Part print with two shaded views. Sizes in mm from the minimum x, y, z corner. A direction names the side the tool comes from. Round coordinates to 2 decimals unless told otherwise and drop trailing zeros. Write each loop counter-clockwise with the first axis right and the second up, starting at its lowest first coordinate (ties: lowest second). Pieces come first, ordered by that corner, then holes.
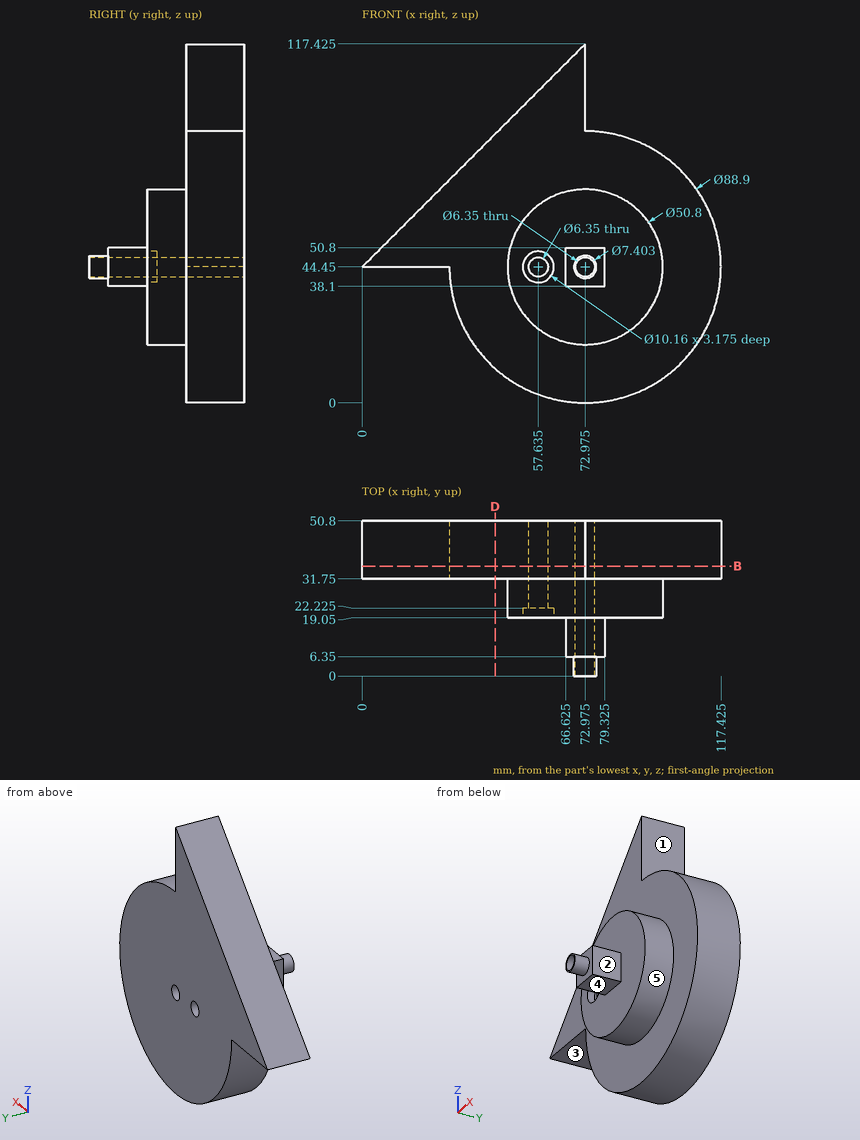
Q1. Drop flat-ended pins along their axis: pin 1 (8 mm diameter, centred on x = 74.5, z = 27, fed in from -Y); pin 2 (10 mm diameter, centred on y = 11.5, z = 47, fed in from +X) (1 decimal); pin 3 (10 mm diameter, centred on x = 70, y = 15, fed in from -Z). Give the stop position or say it passes through.
Values follow:
pin 1: stops at y = 19.05
pin 2: stops at x = 79.3
pin 3: stops at z = 19.05
Q2. Cut at B-B on y = 36. State how many separate pieces and enclosed holes the cut face has.
Values follow:
separate pieces: 1
enclosed holes: 2
Q3. Wall check: L1, parallel to X at y = 25, z = 44; L2, parallel to X at y = 47.5, z = 42 (1 decimal); L3, parallel to Y at x = 90.5, z = 10. Give the ranges that are in metal, low to high.
Values follow:
L1: x = 47.58 to 54.49, 60.78 to 69.83, 76.12 to 98.37
L2: x = 28.6 to 55.6, 59.7 to 71, 75 to 117.4
L3: y = 31.75 to 50.8
Q4. Cut at D-D on x = 43.5. Write the cut outline in (y, z), plus the area to 3 significant figures.
Values follow:
outline: (31.75, 11.18) - (50.8, 11.18) - (50.8, 87.95) - (31.75, 87.95) - close
area: 1,460 mm2
Q5. Which spindle directions (+Z, -Z, +X, -X, +Y, -Y) get a long thin tool onto all of the face, cutting with end or side? Do the marked faces 1, 2, 3, 4 and 5. Say none if no direction does.
Values follow:
face 1: +Z, +X, +Y, -Y
face 2: +Z, -Z, +X, -Y
face 3: -Z, -X, +Y, -Y
face 4: -Z, +X, -X, -Y
face 5: -Y
